Check sheet for the drawn part. Datum: minimum x, y, z corner. Units: mm. Coordinates: 2 decimals unless noted, no trailing zeros. Order: outer loops, then holes, each group sorted by start corner. A loop starts at its lowest first (then second) coordinate and runs counter-clockwise, first axis right, second up.
Q1. Cross-section at C-C, the plane z = 11. Record the boundary of the cut face in (x, y), and give its area (3 significant figures).
Q2. Thickness scan on line 1 (Z direction, x = 11.5, y = 5.75); line 2 (X direction, y = 4.5, z = 57). Record the ranges inside material, lowest first.
Q3. Cross-section at B-B, the plane x = 14.5. Record the boundary of the cut face in (y, z).
Q4. Depth check by flat-ended pin: P1, Ø3, axis at x = 83.5, y = 7, coming from the -Z side; P2, Ø6, axis at y = 9, z = 27.5, coming from the -X side; P3, Ø6, axis at y = 5, z = 58, coming from the +X side. Enter the tip coordinate at first touch or a pass-through.
Q5. Cross-section at A-A, the plane y = 5.5. Record the boundary of the cut face in (x, z).
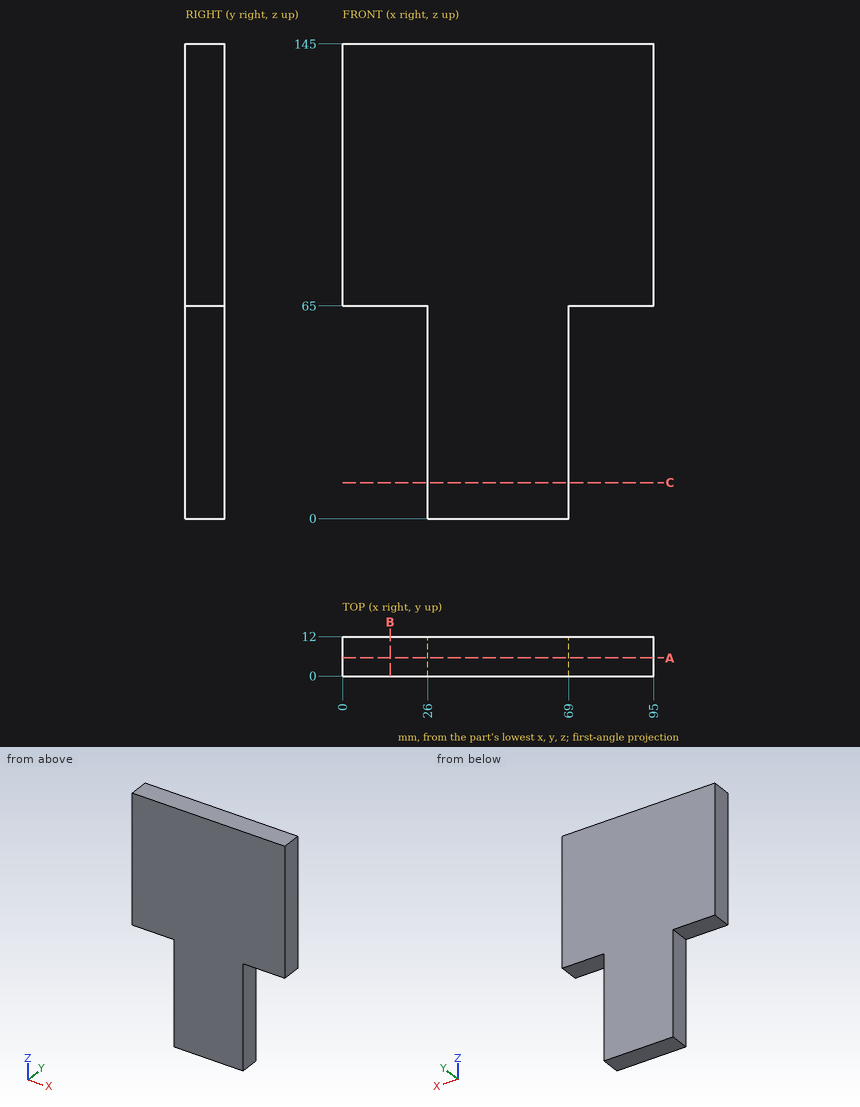
Check values:
1. outline: (26, 0) - (69, 0) - (69, 12) - (26, 12) - close
1. area: 516 mm2
2. line 1: z = 65 to 145
2. line 2: x = 26 to 69
3. outline: (0, 65) - (12, 65) - (12, 145) - (0, 145) - close
4. P1: stops at z = 65
4. P2: stops at x = 26
4. P3: stops at x = 69
5. outline: (0, 65) - (26, 65) - (26, 0) - (69, 0) - (69, 65) - (95, 65) - (95, 145) - (0, 145) - close
